Autodesk Inventor part; units mm, degrees
ref_plane "YZ Plane" through (0, 0, 0) normal (1, 0, 0) x (0, 1, 0)
ref_plane "XZ Plane" through (0, 0, 0) normal (0, 1, 0) x (-1, 0, 0)
ref_plane "XY Plane" through (0, 0, 0) normal (0, 0, 1) x (1, 0, 0)
sketch "スケッチ1" plane through (0, 0, 0) normal (1, 0, 0) x (0, 1, 0)
  circle A0 centre (0, 0) radius 2.5
  line L0 (0, 4.0992) -> (3.55, 2.0496)
  line L1 (3.55, 2.0496) -> (3.55, -2.0496)
  line L2 (3.55, -2.0496) -> (0, -4.0992)
  line L3 (0, -4.0992) -> (-3.55, -2.0496)
  line L4 (-3.55, -2.0496) -> (-3.55, 2.0496)
  line L5 (-3.55, 2.0496) -> (0, 4.0992)
  circle A1 centre (0, 0) radius 5.5
  line L6 (5.5, 0) -> (-5.5, 0) construction
  line L7 (-5.5, 0) -> (-5.5, 30)
  line L8 (-5.5, 30) -> (5.5, 30)
  line L9 (5.5, 30) -> (5.5, 0)
  dimension "d2" = 11
  dimension "d0" = 5
  dimension "d1" = 7.1
  dimension "d3" = 30
extrude "押し出し1" add sketch "スケッチ1" along normal blind 3 contours A1 | A1 L7 L8 L9
extrude "押し出し2" add sketch "スケッチ1" along normal blind 1 contours L0 L1 L2 L3 L4 L5
sketch "スケッチ2" plane through (3, 0, 0) normal (1, 0, 0) x (0, 0, -1)
  circle A0 centre (-10, 0) radius 1.6
  circle A1 centre (-20, 0) radius 1.6
  point P0 (0, 0)
  dimension "d8" = 3.2
  dimension "d9" = 3.2
  dimension "d10" = 10
  dimension "d11" = 10
extrude "押し出し3" cut sketch "スケッチ2" against normal through all
sketch "スケッチ3" plane through (0, 0, 0) normal (-1, 0, 0) x (0, 0, 1)
  circle A0 centre (20, 0) radius 1.6
  circle A1 centre (10, 0) radius 1.6
  line L0 (21.6454, -2.85) -> (18.3546, -2.85)
  line L1 (18.3546, -2.85) -> (16.7091, 0)
  line L2 (16.7091, 0) -> (18.3546, 2.85)
  line L3 (18.3546, 2.85) -> (21.6454, 2.85)
  line L4 (21.6454, 2.85) -> (23.2909, 0)
  line L5 (23.2909, 0) -> (21.6454, -2.85)
  line L6 (11.6454, -2.85) -> (8.3546, -2.85)
  line L7 (8.3546, -2.85) -> (6.7091, 0)
  line L8 (6.7091, 0) -> (8.3546, 2.85)
  line L9 (8.3546, 2.85) -> (11.6454, 2.85)
  line L10 (11.6454, 2.85) -> (13.2909, 0)
  line L11 (13.2909, 0) -> (11.6454, -2.85)
  point P0 (0, 0)
  dimension "d14" = 5.7
extrude "押し出し4" cut sketch "スケッチ3" against normal blind 2
sketch "スケッチ4" plane through (0, 0, 0) normal (-1, 0, 0) x (0, 0, 1)
  line L0 (16.2, 5) -> (-2.2913, 5)
  line L1 (16.2, 5.5) -> (16.2, 5)
  arc A0 (21.2458, 6.2407) -> (21.5454, 6.0705) centre (23.8648, 10.5) ccw
  line L2 (21.5454, 6.0705) -> (16.2, 6.0705)
  line L3 (16.2, 6.0705) -> (16.2, 5.8705)
  line L4 (16.2, 5.8705) -> (21.5454, 5.8705)
  line L5 (21.5454, 5.8705) -> (21.5454, 6.0705)
  arc A1 (0, 5.5) -> (0, -5.5) centre (0, 0) ccw
  line L6 (0, 5.5) -> (30, 5.5)
  point P0 (30, 5.5)
  point P1 (16.2, 5.3)
  dimension "d17" = 0.2
extrude "押し出し5" cut sketch "スケッチ4" against normal through all
sketch "スケッチ5" plane through (0, 0, 0) normal (-1, 0, 0) x (0, 0, 1)
  line L0 (23.2909, 0) -> (21.6454, -2.85)
  line L1 (21.6454, 2.85) -> (23.2909, 0)
  line L2 (30, -5.5) -> (0, -5.5)
  line L3 (21.6454, -5.5) -> (21.6454, 5.5)
  line L4 (16.2, 5.5) -> (30, 5.5)
  line L5 (23.8648, 5.5) -> (23.8648, 5.3)
  line L6 (30, 5.5) -> (30, -5.5)
  line L7 (30, 5.5) -> (16.1, 5.5)
  point P0 (0, 0)
extrude "押し出し6" add sketch "スケッチ5" along normal blind 4 contours L1 L3 L4 L6 L2 L0
sketch "スケッチ7" plane through (-4, 0, 0) normal (-1, 0, 0) x (0, 0, 1)
  line L0 (30, 5.5) -> (21.6454, 5.5)
  line L1 (21.6454, 5.5) -> (21.6454, 2.85)
  line L2 (21.6454, 2.85) -> (23.2909, 0)
  line L3 (23.2909, 0) -> (21.6454, -2.85)
  line L4 (21.6454, -2.85) -> (21.6454, -5.5)
  line L5 (21.6454, -5.5) -> (30, -5.5)
  line L6 (30, -5.5) -> (30, 5.5)
  point P0 (0, 0)
extrude "押し出し7" add sketch "スケッチ7" against normal blind 10
sketch "スケッチ8" plane through (0, -5.5, 0) normal (0, -1, 0) x (1, 0, 0)
  circle A0 centre (3.5, 27) radius 1.6
  circle A1 centre (-1.5, 27) radius 1.6
  line L0 (6, 30) -> (6, 21.6454)
  line L1 (-4, 21.6454) -> (-4, 30)
  line L2 (-4, 30) -> (6, 30)
  point P0 (0, 0)
  dimension "d24" = 3.2
  dimension "d25" = 3.2
  dimension "d26" = 2.5
  dimension "d27" = 2.5
  dimension "d28" = 3
extrude "押し出し8" cut sketch "スケッチ8" against normal through all
equation "\"d11\" = d10"
equation "\"d27\" = d26"
properties part number "hand_finger_inside"
Read the model definition and answer for the solid it produces. Units are mm, in the model's axes. A direction names the side the tool comes from. Coordinates: 2 decimals unless noted, no trailing zeros. Write each loop counter-clockwise with the first axis right and the second up, starting at its lowest first coordinate (ties: lowest second). Pieces come first, ordered by that corner, then holes. Notation, with made-up numbers: (-33.75, 85) - (16.25, 85) arc R17 cw to (16.25, 95) - close; hole circle Ø5 at (-3, -7.5). An arc over 180 degrees is marked (long way). One line per question, with ' | ' between items.
Q1. Find section B-B, the plane y = 2. Write down the section's boundary in (x, z).
Result set:
outline: (-4, 22.14) - (2, 22.14) - (2, 17.86) - (0, 17.86) - (0, 12.14) - (2, 12.14) - (2, 7.86) - (0, 7.86) - (0, 1.5) - (1, 1.5) - (1, 2.94) - (3, 2.94) - (3, 22.14) - (6, 22.14) - (6, 30) - (-4, 30) - close; (0, -5.12) - (3, -5.12) - (3, -2.94) - (1, -2.94) - (1, -1.5) - (0, -1.5) - close; hole circle Ø3.2 at (-1.5, 27); hole circle Ø3.2 at (3.5, 27)
Q2. Determine the mould class of faces 1 (the flat face through (-2, 4, 21.645)), 2 (the flat face through (0, 0, 5)), 3 (the flat face through (0.986, 1.405, 7.52)) for opening direction Z: +Z half, -Z half, draft (parallel to the pull), parting line (faces both ways), or undercut.
Result set:
face 1: -Z half | face 2: draft | face 3: undercut
Q3. Find section C-C, the plane x = 3.5. Write down the section's boundary in (y, z).
Result set:
outline: (-5.5, 21.65) - (-2.85, 21.65) - (0, 23.29) - (2.85, 21.65) - (5.5, 21.65) - (5.5, 25.4) - (-5.5, 25.4) - close; (-5.5, 28.6) - (5.5, 28.6) - (5.5, 30) - (-5.5, 30) - close
Q4. For faces 4 (the flat face through (1, -2.85, 10)), 5 (the flat face through (2, -3.55, 0)), 6 (the flat face through (1, 5, 7)), determine the directions among +Z, -Z, +X, -X, +Y, -Y from which every point of the face is accessible in a straight line to the end or side of a thin tool.
Result set:
face 4: -X | face 5: +X | face 6: -Z, +X, -X, +Y
Q5. Consider L1, parallel to Y at x = 2.2, z = 10; L2, parallel to Z at x = 0.5, y = -0.75; L3, parallel to Z at x = 0.5, y = -0.25. Determine where each line is inside the solid, lowest interval first. Write a range as [from, to].
Result set:
L1: [-5.5, -1.6], [1.6, 5] | L2: [-5.45, -2.38], [2.38, 7.14], [12.86, 17.14], [22.86, 30] | L3: [-5.49, -2.49], [2.49, 6.85], [13.15, 16.85], [23.15, 30]
Q6. Find section D-D, the plane z = 10. Write down the section's boundary in (x, y), plus the area to 3 significant figures.
Result set:
outline: (0, -5.5) - (3, -5.5) - (3, -1.6) - (2, -1.6) - (2, -2.85) - (0, -2.85) - close; (0, 2.85) - (2, 2.85) - (2, 1.6) - (3, 1.6) - (3, 5) - (0, 5) - close | area: 16.9 mm^2
Q7. Find section A-A, the plane z = 27. Write down the section's boundary in (x, y).
Result set:
outline: (-4, -5.5) - (-3.1, -5.5) - (-3.1, 5.5) - (-4, 5.5) - close; (0.1, -5.5) - (1.9, -5.5) - (1.9, 5.5) - (0.1, 5.5) - close; (5.1, -5.5) - (6, -5.5) - (6, 5.5) - (5.1, 5.5) - close
Q8. Each of these flat-tipped pins is pushed along its axis until it touches: P1, Ø3, axis at x = 5, y = 4, coming from the -Z side; P2, Ø1.7, axis at y = -0.5, z = 11, coming from the -X side; P3, Ø2, axis at x = 1.5, y = 3, coming from the -Z side; P4, Ø1.9, axis at y = 0, z = 10, coming from the -X side. Where does it stop, or does it pass through?
Result set:
P1: z = 21.65 | P2: x = 2 | P3: z = -5.12 | P4: through
